```python
from build123d import *

# Parameters (mm, degrees)
SKETCH1_W                = 40
SKETCH1_H                = 19
BOSS_EXTRUDE1_DEPTH      = 39
SKETCH2_W                = 19
SKETCH2_H                = 3
BOSS_EXTRUDE2_DEPTH      = 7.5
BOSS_EXTRUDE2_DEPTH_BACK = 47.5
CUT_EXTRUDE1_DEPTH       = 3
FILLET1_R                = 0.2
SKETCH4_R                = 3
BOSS_EXTRUDE3_DEPTH      = 8
SKETCH6_R                = 6
BOSS_EXTRUDE4_DEPTH      = 3.77


with BuildPart() as part:
    # Sketch1 → Boss-Extrude1 (new body)
    with BuildSketch(Plane(origin=(0, 0, 0), x_dir=(1, 0, 0), z_dir=(0, 1, 0))):
        Rectangle(SKETCH1_W, SKETCH1_H)
    extrude(amount=BOSS_EXTRUDE1_DEPTH)

    # Sketch2 → Boss-Extrude2 (add, two sides)
    with BuildSketch(Plane(origin=(20, 0, 0), x_dir=(0, 0, -1), z_dir=(1, 0, 0))) as boss_extrude2_sk:
        with Locations((0, 31.5)):
            Rectangle(SKETCH2_W, SKETCH2_H)
    extrude(amount=BOSS_EXTRUDE2_DEPTH)
    extrude(boss_extrude2_sk.sketch, amount=-BOSS_EXTRUDE2_DEPTH_BACK)

    # Sketch3 → Cut-Extrude1 (cut)
    with BuildSketch(Plane(origin=(0, 33, 0), x_dir=(1, 0, 0), z_dir=(0, 1, 0))):
        with BuildLine():
            Line((-23.309672477, 2.75), (-25.690327523, 2.75))
            ThreePointArc((-25.690327523, 2.75), (-27.940327523, 5), (-25.690327523, 7.25))
            Line((-25.690327523, 7.25), (-23.309672477, 7.25))
            ThreePointArc((-23.309672477, 7.25), (-21.059672477, 5), (-23.309672477, 2.75))
        make_face()
        with BuildLine():
            Line((-23.309672477, -2.75), (-25.690327523, -2.75))
            ThreePointArc((-25.690327523, -2.75), (-27.940327523, -5), (-25.690327523, -7.25))
            Line((-25.690327523, -7.25), (-23.309672477, -7.25))
            ThreePointArc((-23.309672477, -7.25), (-21.059672477, -5), (-23.309672477, -2.75))
        make_face()
        with BuildLine():
            Line((23.309672477, -2.75), (25.690327523, -2.75))
            ThreePointArc((25.690327523, -2.75), (27.940327523, -5), (25.690327523, -7.25))
            Line((25.690327523, -7.25), (23.309672477, -7.25))
            ThreePointArc((23.309672477, -7.25), (21.059672477, -5), (23.309672477, -2.75))
        make_face()
        with BuildLine():
            Line((23.309672477, 2.75), (25.690327523, 2.75))
            ThreePointArc((25.690327523, 2.75), (27.940327523, 5), (25.690327523, 7.25))
            Line((25.690327523, 7.25), (23.309672477, 7.25))
            ThreePointArc((23.309672477, 7.25), (21.059672477, 5), (23.309672477, 2.75))
        make_face()
    extrude(amount=-CUT_EXTRUDE1_DEPTH, mode=Mode.SUBTRACT)

    # Fillet1
    fillet1_edges = [part.edges().sort_by_distance(p)[0] for p in [
        (27.5, 31.5, 6.337006181),
        (27.5, 31.5, 3.662993819),
        (27.5, 31.5, -3.662993819),
        (27.5, 31.5, -6.337006181),
        (-27.5, 31.5, 3.662993819),
        (-27.5, 31.5, 6.337006181),
        (-27.5, 31.5, -6.337006181),
        (-27.5, 31.5, -3.662993819),
    ]]
    fillet(fillet1_edges, radius=FILLET1_R)

    # Sketch4 → Boss-Extrude3 (add)
    with BuildSketch(Plane(origin=(0, 39, 0), x_dir=(1, 0, 0), z_dir=(0, 1, 0))):
        with Locations((-11, 0)):
            Circle(SKETCH4_R)
    extrude(amount=BOSS_EXTRUDE3_DEPTH)

    # Sketch6 → Boss-Extrude4 (add)
    with BuildSketch(Plane(origin=(0, 39, 0), x_dir=(1, 0, 0), z_dir=(0, 1, 0))):
        with Locations((-11, 0)):
            Circle(SKETCH6_R)
    extrude(amount=BOSS_EXTRUDE4_DEPTH)


solid = part.part
```
Input: part model. Units: mm. Frame: model coordinates. A direction names the side the tool comes from. Round coordinates to 2 decimals unless told otherwise and drop trailing zeros. Order: outer loops, then holes, each group sorted by start corner. A loop starts at its lowest first (then second) coordinate and runs counter-clockwise, first axis right, second up. Notation, with made-up numbers: (-22, 66) - (-10, 66) arc R21 ccw to (-10, 96) - close; hole circle Ø10 at (8, 19.5). An arc over 180 degrees is marked (long way). Answer in a Markdown table with one row per item.
Item 1: Section query A-A (z = 0). Return the cut outline in (x, y), then the cut area to 3 significant figures.
Model answer:
| item | result |
|---|---|
| outline | (-27.5, 30) - (-20, 30) - (-20, 0) - (20, 0) - (20, 30) - (27.5, 30) - (27.5, 33) - (20, 33) - (20, 39) - (-5, 39) - (-5, 42.77) - (-8, 42.77) - (-8, 47) - (-14, 47) - (-14, 42.77) - (-17, 42.77) - (-17, 39) - (-20, 39) - (-20, 33) - (-27.5, 33) - close |
| area | 1,680 mm² |
Item 2: Section query D-D (z = 5). Return the cut outline in (x, y), then the cut area to 3 significant figures.
Model answer:
| item | result |
|---|---|
| outline | (-21.06, 30) - (-20, 30) - (-20, 0) - (20, 0) - (20, 30) - (21.06, 30) - (21.06, 33) - (20, 33) - (20, 39) - (-7.68, 39) - (-7.68, 42.77) - (-14.32, 42.77) - (-14.32, 39) - (-20, 39) - (-20, 33) - (-21.06, 33) - close |
| area | 1,590 mm² |
Item 3: Line query: line 1 (X direction, y = 16, z = 6.5); line 2 (Y direction, x = -10.5, z = 7); line 3 (Y direction, x = 23.5, z = -2.5). Output: solid intervals per line, ascending.
Model answer:
| item | result |
|---|---|
| line 1 | x = -20 to 20 |
| line 2 | y = 0 to 39 |
| line 3 | y = 30 to 33 |
Item 4: Reachability of faces 4 (the cylindrical face through (26.5, 31.5, 7.1)), 5 (the flat face through (-20, 15, 0)), 6 (the flat face through (20, 15, 0)) from +Z, -Z, +X, -X, +Y, -Y: full face, straight path, thin tool, end or side. Return the list, or none.
Model answer:
| item | result |
|---|---|
| face 4 | +Y, -Y |
| face 5 | +Z, -Z, -X, -Y |
| face 6 | +Z, -Z, +X, -Y |
Item 5: Section query B-B (x = -11). Return the cut outline in (y, z).
Model answer:
| item | result |
|---|---|
| outline | (0, -9.5) - (39, -9.5) - (39, -6) - (42.77, -6) - (42.77, -3) - (47, -3) - (47, 3) - (42.77, 3) - (42.77, 6) - (39, 6) - (39, 9.5) - (0, 9.5) - close |
Item 6: Section query C-C (y = 23). Return the cut outline in (x, z), then the cut area to 3 significant figures.
Model answer:
| item | result |
|---|---|
| outline | (-20, -9.5) - (20, -9.5) - (20, 9.5) - (-20, 9.5) - close |
| area | 760 mm² |
Item 7: Mould query, pull axis X, two halves, no side actions, for faces 1 (the flat face through (-24, 32, -2.75)), 2 (the flat face through (0, 19, -9.5)), 3 (the flat face through (-20, 36, 0)). Classes: released by +X, released by -X, zero draft, split by the parting line, or undercut.
Model answer:
| item | result |
|---|---|
| face 1 | undercut |
| face 2 | zero draft |
| face 3 | released by -X |
Item 8: Pin query (flat end, axial travel): pin 1 (3 mm diameter, centred on y = 7, z = 4, fed in from -X); pin 2 (2 mm diameter, centred on x = 24.5, z = -2, fed in from -Y); pin 3 (6 mm diameter, centred on x = 24, z = 2.5, fed in from +Y). Return the tip coordinate at first contact, or that it passes through.
Model answer:
| item | result |
|---|---|
| pin 1 | stops at x = -20 |
| pin 2 | stops at y = 30 |
| pin 3 | stops at y = 33 |
